from build123d import *

# Parameters (mm, degrees)
SKETCH_1_W             = 64
SKETCH_1_H             = 30
EXTRUDE_545_DEPTH      = 13
SKETCH_2_R             = 13.175
CUT_EXTRUDE_683_DEPTH  = 5
CUT_EXTRUDE_START      = -5.5
SKETCH_3_R             = 13.175
CUT_EXTRUDE_807_DEPTH  = 5.5
SKETCH_4_R             = 11.5
CUT_EXTRUDE_897_DEPTH  = 44.462627624
EXTRUDE_START          = 3
SKETCH_8_W             = 64
SKETCH_8_H             = 30
SKETCH_8_R             = 13.175
EXTRUDE_1112_DEPTH     = 3
EXTRUDE_START_2        = 12
SKETCH_9_W             = 10
SKETCH_9_H             = 30
EXTRUDE_1450_DEPTH     = 12
SKETCH_10_R            = 1
CUT_EXTRUDE_1737_DEPTH = 12
SKETCH_11_R            = 1.65
CUT_EXTRUDE_2233_DEPTH = 58.306195128
SKETCH_12_W            = 10
SKETCH_12_H            = 5.4
EXTRUDE_2614_DEPTH     = 2
CUT_EXTRUDE_2853_DEPTH = 3
SKETCH_15_W            = 10
SKETCH_15_H            = 19.2
SKETCH_15_R            = 1
EXTRUDE_3124_DEPTH     = 9
CHAMFER_5_SIZE         = 3
SKETCH_17_W            = 2.9
SKETCH_17_H            = 19.2
EXTRUDE_3548_DEPTH     = 2
SKETCH_16_W            = 7.1
SKETCH_16_H            = 2
CUT_EXTRUDE_3829_DEPTH = 2
SKETCH_18_W            = 4
SKETCH_18_H            = 30
EXTRUDE_3994_DEPTH     = 14
FILLET_4_R             = 3
CHAMFER_7_SIZE         = 1


with BuildPart() as part:
    # Эскиз1 → Extrude 545 (new body)
    with BuildSketch(Plane(origin=(0, 0, 0), x_dir=(1, 0, 0), z_dir=(0, 1, 0))):
        with Locations((8, 0)):
            Rectangle(SKETCH_1_W, SKETCH_1_H)
    extrude(amount=EXTRUDE_545_DEPTH)

    # Эскиз2 → Cut-Extrude 683 (cut)
    with BuildSketch(Plane(origin=(0, 13, 0), x_dir=(1, 0, 0), z_dir=(0, 1, 0))):
        with Locations(Location((0, 0, 0), (0, 0, 270))):
            Circle(SKETCH_2_R)
    extrude(amount=-CUT_EXTRUDE_683_DEPTH, mode=Mode.SUBTRACT)

    # Эскиз3 → Cut-Extrude 807 (cut)
    with BuildSketch(Plane.XZ.offset(CUT_EXTRUDE_START)):
        with Locations(Location((0, 0, 0), (0, 0, 90))):
            Circle(SKETCH_3_R)
    extrude(amount=CUT_EXTRUDE_807_DEPTH, mode=Mode.SUBTRACT)

    # Эскиз4 → Cut-Extrude 897 (cut, through all)
    with BuildSketch(Plane(origin=(0, 8, 0), x_dir=(1, 0, 0), z_dir=(0, 1, 0))):
        with Locations(Location((0, 0, 0), (0, 0, 270))):
            Circle(SKETCH_4_R)
    extrude(amount=-CUT_EXTRUDE_897_DEPTH, mode=Mode.SUBTRACT)

    # Эскиз8 → Extrude 1112 (add)
    with BuildSketch(Plane(origin=(0, 13, 0), x_dir=(1, 0, 0), z_dir=(0, 1, 0)).offset(EXTRUDE_START)):
        with Locations((8, 0)):
            Rectangle(SKETCH_8_W, SKETCH_8_H)
        with Locations(Location((0, 0, 0), (0, 0, 270))):
            Circle(SKETCH_8_R, mode=Mode.SUBTRACT)
    extrude(amount=-EXTRUDE_1112_DEPTH)

    # Эскиз9 → Extrude 1450 (add)
    with BuildSketch(Plane(origin=(0, 16, 0), x_dir=(1, 0, 0), z_dir=(0, 1, 0)).offset(EXTRUDE_START_2)):
        with BuildLine():
            Line((-20, 15), (-10, 15))
            Line((-10, 15), (-10, 8.577914956))
            ThreePointArc((-10, 8.577914956), (-13.175, 0), (-10, -8.577914956))
            Line((-10, -8.577914956), (-10, -15))
            Line((-10, -15), (-20, -15))
            Line((-20, -15), (-20, 15))
        make_face()
        with Locations((35, 0)):
            Rectangle(SKETCH_9_W, SKETCH_9_H)
    extrude(amount=-EXTRUDE_1450_DEPTH)

    # Эскиз10 → Cut-Extrude 1737 (cut)
    with BuildSketch(Plane(origin=(0, 28, 0), x_dir=(1, 0, 0), z_dir=(0, 1, 0))):
        with Locations(Location((-14, 5, 0), (0, 0, 270))):
            Circle(SKETCH_10_R)
        with Locations(Location((-14, -5, 0), (0, 0, 270))):
            Circle(SKETCH_10_R)
        with Locations(Location((34, -5, 0), (0, 0, 270))):
            Circle(SKETCH_10_R)
        with Locations(Location((34, 5, 0), (0, 0, 270))):
            Circle(SKETCH_10_R)
    extrude(amount=-CUT_EXTRUDE_1737_DEPTH, mode=Mode.SUBTRACT)

    # Эскиз11 → Cut-Extrude 2233 (cut, through all)
    with BuildSketch(Plane.XY.offset(15)):
        with Locations((-18, 8)):
            Circle(SKETCH_11_R)
        with Locations((34, 8)):
            Circle(SKETCH_11_R)
    extrude(amount=-CUT_EXTRUDE_2233_DEPTH, mode=Mode.SUBTRACT)

    # Эскиз12 → Extrude 2614 (add)
    with BuildSketch(Plane(origin=(0, 28, 0), x_dir=(1, 0, 0), z_dir=(0, 1, 0))):
        with Locations((-15, 12.3)):
            Rectangle(SKETCH_12_W, SKETCH_12_H)
        with Locations((-15, -12.3)):
            Rectangle(SKETCH_12_W, SKETCH_12_H)
        with Locations((35, -12.3)):
            Rectangle(SKETCH_12_W, SKETCH_12_H)
        with Locations((35, 12.3)):
            Rectangle(SKETCH_12_W, SKETCH_12_H)
    extrude(amount=EXTRUDE_2614_DEPTH)

    # Эскиз14 → Cut-Extrude 2853 (cut)
    with BuildSketch(Plane(origin=(0, 16, 0), x_dir=(1, 0, 0), z_dir=(0, 1, 0))):
        with BuildLine():
            Line((-10, 15), (-10, 8.577914956))
            ThreePointArc((-10, 8.577914956), (13.175, 0), (-10, -8.577914956))
            Line((-10, -8.577914956), (-10, -15))
            Line((-10, -15), (30, -15))
            Line((30, -15), (30, 15))
            Line((30, 15), (-10, 15))
        make_face()
    extrude(amount=-CUT_EXTRUDE_2853_DEPTH, mode=Mode.SUBTRACT)

    # Эскиз15 → Extrude 3124 (add)
    with BuildSketch(Plane(origin=(0, 28, 0), x_dir=(1, 0, 0), z_dir=(0, 1, 0))):
        with Locations((-15, 0)):
            Rectangle(SKETCH_15_W, SKETCH_15_H)
        with Locations(Location((-14, 5, 0), (0, 0, 270))):
            Circle(SKETCH_15_R, mode=Mode.SUBTRACT)
        with Locations(Location((-14, -5, 0), (0, 0, 270))):
            Circle(SKETCH_15_R, mode=Mode.SUBTRACT)
    extrude(amount=-EXTRUDE_3124_DEPTH)

    # Фаска5
    chamfer_5_edges = [part.edges().sort_by_distance(p)[0] for p in [
        (-10, 19, 0),
    ]]
    chamfer(chamfer_5_edges, length=CHAMFER_5_SIZE)

    # Эскиз17 → Extrude 3548 (add)
    with BuildSketch(Plane(origin=(0, 28, 0), x_dir=(1, 0, 0), z_dir=(0, 1, 0))):
        with Locations((-18.55, 0)):
            Rectangle(SKETCH_17_W, SKETCH_17_H)
        with Locations((38.55, 0)):
            Rectangle(SKETCH_17_W, SKETCH_17_H)
    extrude(amount=EXTRUDE_3548_DEPTH)

    # Эскиз16 → Cut-Extrude 3829 (cut)
    with BuildSketch(Plane(origin=(0, 28, 0), x_dir=(1, 0, 0), z_dir=(0, 1, 0))):
        with Locations((-13.55, 0)):
            Rectangle(SKETCH_16_W, SKETCH_16_H)
        with Locations((33.55, 0)):
            Rectangle(SKETCH_16_W, SKETCH_16_H)
    extrude(amount=-CUT_EXTRUDE_3829_DEPTH, mode=Mode.SUBTRACT)

    # Эскиз18 → Extrude 3994 (add)
    with BuildSketch(Plane(origin=(0, 16, 0), x_dir=(1, 0, 0), z_dir=(0, 1, 0))):
        with Locations((-22, 0)):
            Rectangle(SKETCH_18_W, SKETCH_18_H)
    extrude(amount=EXTRUDE_3994_DEPTH)

    # Скругление4
    fillet_4_edges = [part.edges().sort_by_distance(p)[0] for p in [
        (30, 13, 0),
        (-10, 13, 11.788957478),
        (-10, 13, -11.788957478),
    ]]
    fillet(fillet_4_edges, radius=FILLET_4_R)

    # Фаска7
    chamfer_7_edges = [part.edges().sort_by_distance(p)[0] for p in [
        (-17, 30, -15),
        (-17, 30, 15),
        (40, 30, 0),
        (35, 30, 15),
        (35, 30, -15),
        (-24, 30, 0),
    ]]
    chamfer(chamfer_7_edges, length=CHAMFER_7_SIZE)


solid = part.part
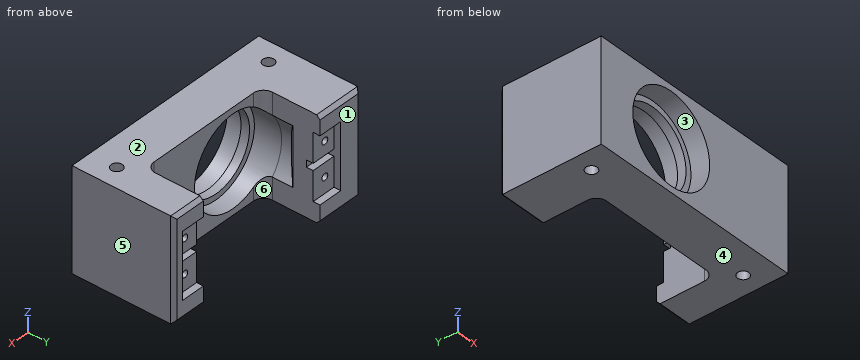
Check sheet for the modelled part. Datum: model origin and axes. Units: mm. Face numbers are marked on the shaded views. A direction names the side the tool comes from. Round coordinates to 2 decimals unless told otherwise and drop trailing zeros. Order: outer loops, then holes, each group sorted by start corner. A loop starts at its lowest first (then second) coordinate and runs counter-clockwise, first axis right, second up. Notation, with made-up numbers: M 16,82 L 43,82 A28 ccw 43,116 Z; hole C 42.25,37 d8. An arc over 180 degrees is marked long. One line per item, written item: value. Start each with the question number.
1. Scan lines: line 1 along X through (y, z) = (24, -5); line 2 along X through (y, z) = (22.75, 12.5); line 3 along X through (y, z) = (16.75, 5). Record each from-to range of solid material in increasing order.
2. Section check A-A on y = 27.25. Enter the section's corners in (x, z).
3. Gauge pin test, flat ends, axial feed: P1, Ø1.5, axis at x = 30.5, z = 0, coming from the +Y side; P2, Ø3.5, axis at x = 34.5, z = 4, coming from the +Y side; P3, Ø1.8, axis at x = 34, z = -5, coming from the +Y side. Record the tip position at first contact, or that the pin passes through.
4. Access from +Z, -Z, +X, -X, +Y, -Y to the whole of each face (thin tool, end or side, straight path). Record for the marked faces 5 and 6.
5. Section check D-D on y = 11. Enter the section's corners in (x, z) (3 decimals), and give its area (3 significant figures).
6. Section check B-B on z = 0. Give the number of separate pieces and of enclosed holes in the cut face, and give its area (3 significant figures).
7. Section check C-C on x = -18. Enter the section's corners in (y, z), and give its area (3 significant figures).
8. Release check for a two-part mould opening along Z. For the marked faces 1, 2, 3 and 4 record: released by +Z, released by -Z, zero draft, split by the parting line, or undercut.
Results found:
1. line 1: -24 to -15, -13 to -10, 30 to 33, 35 to 40
1. line 2: -24 to -10, 30 to 40
1. line 3: -24 to -15, -13 to -12.19, 30 to 33, 35 to 40
2. outline: M -24,-15 L -10,-15 L -10,-1 L -17.1,-1 L -17.1,1 L -10,1 L -10,15 L -24,15 Z; M 30,-15 L 40,-15 L 40,15 L 30,15 L 30,1 L 37.1,1 L 37.1,-1 L 30,-1 Z; hole C -14,-5 d2; hole C -14,5 d2; hole C 34,-5 d2; hole C 34,5 d2
3. P1: y = 26
3. P2: y = 28
3. P3: y = 16
4. face 5: +Z, -Z, +X, +Y, -Y
4. face 6: +Z, -Z, +Y
5. outline: M -24,-15 L 40,-15 L 40,15 L -24,15 Z; hole C 0,0 d26.35
5. area: 1,370 mm^2
6. separate pieces: 2
6. enclosed holes: 2
6. area: 809 mm^2
7. outline: M 0,-15 L 6.35,-15 L 6.35,15 L 0,15 Z; M 9.65,-15 L 29,-15 L 30,-14 L 30,14 L 29,15 L 9.65,15 Z
7. area: 800 mm^2
8. face 1: zero draft
8. face 2: released by +Z
8. face 3: undercut
8. face 4: released by -Z
